```python
from build123d import *

# Parameters (mm, degrees)
F1_DEPTH = 6.35
F2_R     = 6.35
F3_DEPTH = 25.4
F6_START = 35.56
F6_DEPTH = 27.94
F7_R     = 5.08
F8_R     = 4.445
F9_DEPTH = 25.4
F10_R    = 5.08
F11_SIZE = 1.016


with BuildPart() as f1:
    # F0 (on Top) → F1 (new body)
    with BuildSketch(Plane.XY):
        Polygon((38.1, 25.4), (0, 25.4), (-38.1, 25.4), (-38.1, 0), (-38.1, -25.4), (0, -25.4), (38.1, -25.4), (38.1, 0), align=None)
    extrude(amount=F1_DEPTH)

    # F2 (on face) → F3 (cut)
    with BuildSketch(Plane.XY.offset(6.35)):
        with BuildLine():
            Line((-19.05, 0), (-19.05, 10.7293000911))
            ThreePointArc((-19.05, 10.7293000911), (-24.13, 15.8093000911), (-29.21, 10.7293000911))
            Line((-29.21, 10.7293000911), (-29.21, 0))
            Line((-29.21, 0), (-29.21, -10.7293000911))
            ThreePointArc((-29.21, -10.7293000911), (-24.13, -15.8093000911), (-19.05, -10.7293000911))
            Line((-19.05, -10.7293000911), (-19.05, 0))
        make_face()
        with Locations((26.67, -13.97)):
            Circle(F2_R)
    extrude(amount=-F3_DEPTH, mode=Mode.SUBTRACT)

    # F5 (on face) → F6 (join)
    with BuildSketch(Plane(origin=(-31.75, -31.75, 0), x_dir=(-0.7071067812, 0.7071067812, 0), z_dir=(0.7071067812, 0.7071067812, 0)).offset(F6_START)):
        Polygon((-7.62, 6.35), (0, 6.35), (7.62, 38.4787410273), (0, 38.4787410273), align=None)
    extrude(amount=F6_DEPTH)

    # F7
    f7_edges = [f1.edges().sort_by_distance(p)[0] for p in [
        (-9.29936, -3.911206, 38.478741),
        (10.457204, 15.845357, 38.478741),
    ]]
    fillet(f7_edges, radius=F7_R)

    # F8 (on face) → F9 (cut)
    with BuildSketch(Plane(origin=(6.1094258432, -6.1094258432, 2.0491637233), x_dir=(0.6523063877, 0.7256908563, 0.2187902138), z_dir=(0.6880209162, -0.6880209162, 0.2307692308))):
        with Locations((10.9869780004, 28.0684145883)):
            Circle(F8_R)
    extrude(amount=-F9_DEPTH, mode=Mode.SUBTRACT)

    # F10
    f10_edges = [f1.edges().sort_by_distance(p)[0] for p in [
        (38.1, -25.4, 3.175),
        (38.1, 25.4, 3.175),
        (-38.1, -25.4, 3.175),
        (-38.1, 25.4, 3.175),
    ]]
    fillet(f10_edges, radius=F10_R)

    # F11
    f11_edges = [f1.edges().sort_by_distance(p)[0] for p in [
        (0, -25.4, 6.35),
        (38.1, 0, 6.35),
        (36.612102, -23.912102, 6.35),
        (36.612102, 23.912102, 6.35),
        (0, 25.4, 6.35),
        (-36.612102, 23.912102, 6.35),
        (-38.1, 0, 6.35),
        (-36.612102, -23.912102, 6.35),
    ]]
    chamfer(f11_edges, length=F11_SIZE)


solid = f1.part
```
Can you work these out from the model? Positions are in its coordinate system, mm. A direction names the side the tool comes from. Give positions to 0.01 mm unless a question says otherwise; leave off trailing zeros. Loops run counter-clockwise (first coordinate to the right, second up) from the corner with the lowest first, then second, coordinate; pieces in that order, holes last. Notation, with made-up numbers: M 52,3.25 L 70,3.25 A36 cw 70,38.25 Z; hole C -26.75,68.5 d3. An arc over 180 degrees is marked long. Use CSV: the item, a comma, the result in double quotes. Start each with the question number.
1. Imagine slicing it at C-C, the plane y = -13.97. Write out the boundary of the cut face in (x, z), plus the area to 3 significant figures.
2. Imagine slicing it at B-B, the plane x = -24.13. Write out the boundary of the cut face in (y, z), plus the area to 3 significant figures.
3. For P1, Ø1, axis at x = 16, y = 14.5, coming from the +Z side; P2, Ø1, axis at x = 20, z = 6.5, coming from the +Y side; P3, Ø8, axis at y = -11, z = 31, coming from the -X side, each with a flat end and sliding along its axis, tell me the tip position at first contact or that it passes through.
4. Imagine slicing it at D-D, the plane z = 17. Write out the boundary of the cut face in (x, y), plus the area to 3 significant figures.
5. Imagine slicing it at A-A, the plane x = 26.67. Write out the boundary of the cut face in (y, z), plus the area to 3 significant figures.
6. If I drill on L1, parallel to Y at x = 26.67, z = 4.5; L2, parallel to X at y = -13, z = 2; L3, parallel to Z at x = -19, y = -22.5, over which ranges is the centre line in solid material (lowest first)?
7. On a 3-axis mill with a long thin cutter (end or side, diameter ignored), from which of +Z, -Z, +X, -X, +Y, -Y can I reach the whole of each face in a straight line? I mean faces 1 (the face through (-24.24, -15.81, 3.22)), 2 (the face through (-6.11, -7.1, 20.06)), 3 (the face through (13.6, 12.7, 20.1)). Say none if no direction works.
8. If we mould it in two halves opening along Y, with no side actions, what happens to faces 4 (the face through (-36.572, 23.951, 2.704)), 5 (the face through (0, -25.4, 3)), 6 (the face through (-24.02, 15.81, 3.22))? For each: released by +Y, released by -Y, zero draft, split by the parting line, or undercut.
Response values:
1,outline,"M -38.1,0 L -28.04,0 L -28.04,6.35 L -37.08,6.35 L -38.1,5.33 Z; M -20.22,0 L 20.32,0 L 20.32,6.35 L -20.22,6.35 Z; M 33.02,0 L 38.1,0 L 38.1,5.33 L 37.08,6.35 L 33.02,6.35 Z"
1,area,"353 mm^2"
2,outline,"M -25.4,0 L -15.81,0 L -15.81,6.35 L -24.38,6.35 L -25.4,5.33 Z; M 15.81,0 L 25.4,0 L 25.4,5.33 L 24.38,6.35 L 15.81,6.35 Z"
2,area,"121 mm^2"
3,P1,"z = 6.35"
3,P2,"y = 24.73"
3,P3,"x = -6.21"
4,outline,"M -8.39,-4.82 L -3,-10.21 L 16.75,9.55 L 11.37,14.94 Z"
4,area,"213 mm^2"
5,outline,"M -25.4,0 L -20.32,0 L -20.32,6.35 L -24.38,6.35 L -25.4,5.33 Z; M -7.62,0 L 25.4,0 L 25.4,5.33 L 24.38,6.35 L -7.62,6.35 Z"
5,area,"241 mm^2"
6,L1,"-25.4 to -20.32, -7.62 to 25.4"
6,L2,"-38.1 to -28.67, -19.59 to 20.39, 32.95 to 38.1"
6,L3,"0 to 6.35"
7,face 1,"+Z, -Z"
7,face 2,"+Z, -X, -Y"
7,face 3,"+Z, +X, +Y"
8,face 4,"released by +Y"
8,face 5,"released by -Y"
8,face 6,"undercut"
